from build123d import *

# Parameters (mm, degrees)
F0_W            = 9
F0_H            = 11
F3_DEPTH        = 12
F3_COPIES_COUNT = 10
F5_DEPTH        = 25
F6_R            = 3.9
F7_DEPTH        = 4


# Not quite as in the source:
# - a pattern or mirror of a feature is missing from the dataset's text; its kind, count and spacing are read off the source's solid


with BuildPart() as f1:
    # F0 (on Front) → F1 (revolve)
    with BuildSketch(Plane.XZ):
        with Locations((-4.5, 5.5)):
            Rectangle(F0_W, F0_H)
    revolve(axis=Axis((0, 0, 5.5), (0, 0, 1)))

    # F2 (on face) → F3 (cut)
    with BuildSketch(Plane.XY.offset(11)):
        with BuildLine():
            ThreePointArc((-0.495692908, 6.4810715581), (0, 6.5), (0.495692908, 6.4810715581))
            ThreePointArc((0.495692908, 6.4810715581), (0.7861862119, 6.5479757718), (0.9869770252, 6.7683063932))
            Line((0.9869770252, 6.7683063932), (1.7567161864, 8.4190173512))
            ThreePointArc((1.7567161864, 8.4190173512), (1.9988344627, 8.6609895549), (2.3398624375, 8.6905145862))
            ThreePointArc((2.3398624375, 8.6905145862), (0, 9), (-2.3398624375, 8.6905145862))
            ThreePointArc((-2.3398624375, 8.6905145862), (-1.9988344627, 8.6609895549), (-1.7567161864, 8.4190173512))
            Line((-1.7567161864, 8.4190173512), (-0.9869770252, 6.7683063932))
            ThreePointArc((-0.9869770252, 6.7683063932), (-0.7861862119, 6.5479757718), (-0.495692908, 6.4810715581))
        make_face()
    f3 = extrude(amount=-F3_DEPTH, mode=Mode.SUBTRACT)

    # F3_copies: F3 ×10 about axis
    f3_copies_axis = Axis((0, 0, 0), (0, 0, 1))
    for i in range(1, F3_COPIES_COUNT):
        add(f3.rotate(f3_copies_axis, i * 360 / F3_COPIES_COUNT), mode=Mode.SUBTRACT)

    # F4 (on face) → F5 (cut)
    with BuildSketch(Plane.XY.offset(11)):
        with BuildLine():
            Line((-1.65, -2.2), (1.65, -2.2))
            ThreePointArc((1.65, -2.2), (0, 2.75), (-1.65, -2.2))
        make_face()
    extrude(amount=-F5_DEPTH, mode=Mode.SUBTRACT)

    # F6 (on face) → F7 (join)
    with BuildSketch(Plane(origin=(0, 0, 0), x_dir=(1, 0, 0), z_dir=(0, 0, -1))):
        Circle(F6_R)
        with BuildLine():
            ThreePointArc((1.65, 2.2), (0, -2.75), (-1.65, 2.2))
            Line((-1.65, 2.2), (1.65, 2.2))
        make_face(mode=Mode.SUBTRACT)
    extrude(amount=F7_DEPTH)


solid = f1.part
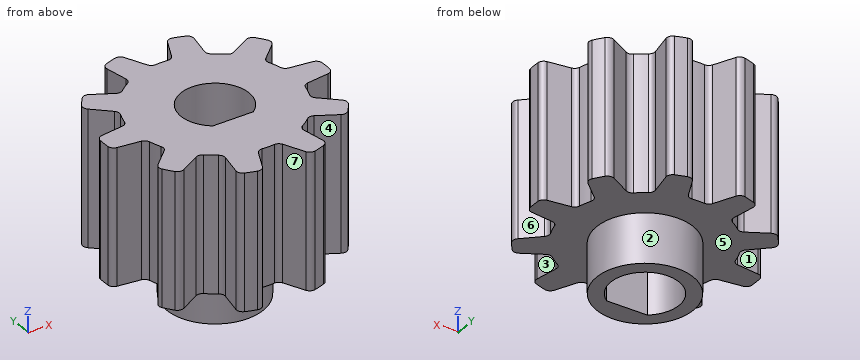
The listing builds one solid part. Answer for the finished solid, in the listing's coordinates (mm). Face numbers are marked on the shaded views. A direction names the side the tool comes from. Round coordinates to 2 decimals unless told otherwise and drop trailing zeros. Loops run counter-clockwise (first coordinate to the right, second up) from the corner with the lowest first, then second, coordinate; pieces in that order, holes last. Notation, with made-up numbers: M 74.25,-40 L 104.25,-40 A15 ccw 104.25,-23 Z; hole C 25,18 d9. An arc over 180 degrees is marked long. Write each question's results on one line, items separated by ' | '. Start each with the question number.
1) Find section D-D on y = -2.75. Write down the section's boundary in (x, z), plus the area to 3 significant figures.
2) Which of the six approach directions +Z, -Z, +X, -X, +Y, -Y give full straight-line access (tool end or side, diameter ignored) to the marked faces 1, 2, 3 and 4?
3) Each of these flat-tipped pins is pushed along its axis until it touches: pin 1 (2 mm diameter, centred on y = 3.5, z = 2, fed in from -X); pin 2 (1.5 mm diameter, centred on y = 3, z = 0.5, fed in from +X); pin 3 (1.5 mm diameter, centred on x = -3.5, y = -6, fed in from -Z); pin 4 (3 mm diameter, centred on y = 5.5, z = -2, fed in from -X). Where does it stop, or does it pass through?
4) Straight lines are drawn through the part: probe 1 along Y at (x, z) = (0, 3.25); probe 2 along X at (y, z) = (0, 4.25); probe 3 along X at (y, z) = (0, -0.75). For each, find the intervals that lie inside material, in ascending order.
5) Find section A-A on y = 0. Write down the section's boundary in (x, z).
6) Find section C-C on z = -1.25. Write down the section's boundary in (x, y), plus the area to 3 significant figures.
7) Determine the mould class of the marked faces 5, 6 and 7 for opening direction Y: pulls with the +Y half, pulls with the -Y half, needs draft (parallel to the pull), parting line crosses it, or undercut.
8) Find section B-B on x = 0. Write down the section's boundary in (y, z), plus the area to 4 significant figures.
Final values:
1) outline: M -5.98,0 L -2.77,0 L -2.77,-4 L 2.77,-4 L 2.77,0 L 5.98,0 L 5.98,11 L -5.98,11 Z | area: 154 mm²
2) face 1: +Z, -Z, -X | face 2: -Z | face 3: +Z, -Z, +X | face 4: +Z, -Z, -Y
3) pin 1: x = -7.6 | pin 2: x = 6.9 | pin 3: z = 0 | pin 4: through
4) probe 1: -6.5 to -2.2, 2.75 to 6.5 | probe 2: -9 to -2.75, 2.75 to 9 | probe 3: -3.9 to -2.75, 2.75 to 3.9
5) outline: M -9,0 L -3.9,0 L -3.9,-4 L -2.75,-4 L -2.75,11 L -9,11 Z; M 2.75,-4 L 3.9,-4 L 3.9,0 L 9,0 L 9,11 L 2.75,11 Z
6) outline: C 0,0 d7.8; hole M -1.65,-2.2 L 1.65,-2.2 A2.75 ccw long Z | area: 25.3 mm²
7) face 5: needs draft | face 6: undercut | face 7: pulls with the -Y half
8) outline: M -6.5,0 L -3.9,0 L -3.9,-4 L -2.2,-4 L -2.2,11 L -6.5,11 Z; M 2.75,-4 L 3.9,-4 L 3.9,0 L 6.5,0 L 6.5,11 L 2.75,11 Z | area: 99.95 mm²
